Verification items for the finished model (mm, model axes). Face numbers are marked on the shaded views. A direction names the side the tool comes from. Coordinates: 2 decimals unless noted, no trailing zeros. Loops run counter-clockwise (first coordinate to the right, second up) from the corner with the lowest first, then second, coordinate; pieces in that order, holes last. Notation, with made-up numbers: (-1.5, -19.75) - (21.5, -19.75) arc R24 ccw to (21.5, 2.25) - close; hole circle Ø2 at (-33, 10.25). An arc over 180 degrees is marked (long way). Answer as CSV lines item,"result". Start each with the question number.
1. Gauge pin test, flat ends, axial feed: P1, Ø11, axis at x = 14.5, y = 75, coming from the +Z side; P2, Ø6, axis at x = 51.5, z = 40, coming from the +Y side; P3, Ø11, axis at y = 87, z = 4, coming from the -X side. Record the tip position at first contact, or that the pin passes through.
2. Cross-section at B-B (y = 54). Enter the section's corners in (x, z), plus the area to 3 significant figures.
3. Cross-section at A-A (x = 60). State how many separate pieces and enclosed holes the cut face has, plus the area to 3 significant figures.
4. Material ranges on line 1 (X direction, y = 85, z = -20); line 2 (X direction, y = 11, z = -58); line 3 (Z direction, x = 66, y = 67), recorded low to high. Write a range as [from, to].
5. Cross-section at C-C (z = 38). Enter the section's corners in (x, y).
6. Release check for a two-part mould opening along X. For the marked faces 5, 6 and 7 record: pulls with the +X half, pulls with the -X half, needs draft (parallel to the pull), parting line crosses it, or undercut.
7. Set-up check for the marked faces 1, 2, 3 and 4: record each of +Z, -Z, +X, -X, +Y, -Y from which the full face is reachable in a straight line by a thin tool's end or side.
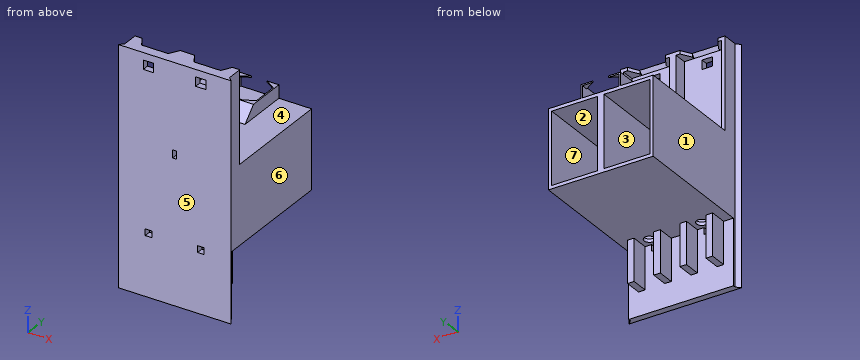
```python
from build123d import *

# Parameters (mm, degrees)
SKETCH1_W                                 = 80
SKETCH1_H                                 = 60
BOSS_EXTRUDE1_DEPTH                       = 100
CUT_EXTRUDE1_START                        = 5
SKETCH2_W                                 = 35
SKETCH2_H                                 = 55
CUT_EXTRUDE1_DEPTH                        = 95
SKETCH3_W                                 = 80
SKETCH3_H                                 = 5
BOSS_EXTRUDE2_DEPTH                       = 70
BOSS_EXTRUDE3_DEPTH                       = 10
SKETCH5_W                                 = 20
SKETCH5_H                                 = 2.5
CUT_EXTRUDE2_DEPTH                        = 7.5
SKETCH6_W                                 = 35
SKETCH6_H                                 = 12
CUT_EXTRUDE4_DEPTH                        = 57.5
CUT_EXTRUDE6_REACH                        = 184.483
SKETCH7_R                                 = 4
SKETCH9_W                                 = 80
SKETCH9_H                                 = 50
BOSS_EXTRUDE4_DEPTH                       = 5
SKETCH13_W                                = 8
SKETCH13_H                                = 7
CUT_EXTRUDE8_BUTTON_HOLES_DEPTH           = 166.90660023
BOSS_EXTRUDE5_OLED_MOUNT_DEPTH            = 10
BOSS_EXTRUDE6_OLED_MOUNT_DEPTH            = 1
BOSS_EXTRUDE7_START                       = -2.5
BOSS_EXTRUDE7_OLED_MOUNT_DEPTH            = 1
BOSS_EXTRUDE8_OLED_MOUNT_DEPTH            = 1
BOSS_EXTRUDE13_OLED_MOUNT_SUPPORT_DEPTH   = 30
CUT_EXTRUDE9_OLED_CABLE_DEPTH             = 10
CUT_EXTRUDE9_OLED_CABLE_DEPTH_BACK        = 154.430766146
SKETCH18_W                                = 3
SKETCH18_H                                = 6
BOSS_EXTRUDE12_OLED_CABLE_GUIDE_REACH     = 162.39
SKETCH20_W                                = 5
SKETCH20_H                                = 5
CUT_EXTRUDE10_SOLENOID_WIRE_HOLE_DEPTH    = 166.90660023
SKETCH21_W                                = 5
SKETCH21_H                                = 32
BOSS_EXTRUDE9_SOLENOID_SIDE_SUPPORT_DEPTH = 13
CHAMFER3_THUMB_SIZE                       = 2.5
CHAMFER5_THUMB_SIZE                       = 4.5
CHAMFER5_THUMB_SIZE2                      = 7.794228634
CHAMFER5_THUMB_PART_2_SIZE                = 4.5
CHAMFER5_THUMB_PART_2_SIZE2               = 7.794228634
CHAMFER5_THUMB_PART_3_SIZE                = 4.5
CHAMFER5_THUMB_PART_3_SIZE2               = 7.794228634
BOSS_EXTRUDE5_GUIDE_DEPTH                 = 180
SKETCH49_W                                = 5
SKETCH49_H                                = 5
BOSS_EXTRUDE14_DEPTH                      = 5
CHAMFER8_SIZE                             = 5


with BuildPart() as part:
    # Sketch1 → Boss-Extrude1 (new body)
    with BuildSketch(Plane(origin=(0, 0, 0), x_dir=(1, 0, 0), z_dir=(0, 1, 0))):
        with Locations((40, 30)):
            Rectangle(SKETCH1_W, SKETCH1_H)
    extrude(amount=BOSS_EXTRUDE1_DEPTH)

    # Sketch2 → Cut-Extrude1 (cut)
    with BuildSketch(Plane(origin=(0, 0, 0), x_dir=(1, 0, 0), z_dir=(0, 1, 0)).offset(CUT_EXTRUDE1_START)):
        with Locations((20, 30)):
            Rectangle(SKETCH2_W, SKETCH2_H)
        with Locations((60, 30)):
            Rectangle(SKETCH2_W, SKETCH2_H)
    extrude(amount=CUT_EXTRUDE1_DEPTH, mode=Mode.SUBTRACT)

    # Sketch3 → Boss-Extrude2 (add)
    with BuildSketch(Plane.XY):
        with Locations((40, 2.5)):
            Rectangle(SKETCH3_W, SKETCH3_H)
    extrude(amount=BOSS_EXTRUDE2_DEPTH)

    # Sketch4 → Boss-Extrude3 (add)
    with BuildSketch(Plane(origin=(0, 5, 0), x_dir=(1, 0, 0), z_dir=(0, 1, 0))):
        Polygon((80, 0), (77.5, 0), (77.5, -67.5), (42.5, -67.5), (42.5, 0), (37.5, 0), (37.5, -67.5), (2.5, -67.5), (2.5, 0), (0, 0), (0, -70), (80, -70), align=None)
    extrude(amount=BOSS_EXTRUDE3_DEPTH)

    # Sketch5 → Cut-Extrude2 (cut)
    with BuildSketch(Plane(origin=(0, 15, 0), x_dir=(1, 0, 0), z_dir=(0, 1, 0))):
        with Locations((20, -68.75)):
            Rectangle(SKETCH5_W, SKETCH5_H)
        with Locations((60, -68.75)):
            Rectangle(SKETCH5_W, SKETCH5_H)
    extrude(amount=-CUT_EXTRUDE2_DEPTH, mode=Mode.SUBTRACT)

    # Sketch6 → Cut-Extrude4 (cut)
    with BuildSketch(Plane.XY):
        with Locations((20, 11)):
            Rectangle(SKETCH6_W, SKETCH6_H)
        with Locations((60, 11)):
            Rectangle(SKETCH6_W, SKETCH6_H)
    extrude(amount=-CUT_EXTRUDE4_DEPTH, mode=Mode.SUBTRACT)

    # Sketch7 → Cut-Extrude6 (cut, up to next)
    with BuildSketch(Plane(origin=(0, 0, -60), x_dir=(-1, 0, 0), z_dir=(0, 0, -1)), mode=Mode.PRIVATE) as cut_extrude6_sk1:
        with Locations((-20, 11.5)):
            Circle(SKETCH7_R)
    cut_extrude6_tool1 = extrude(cut_extrude6_sk1.sketch, amount=-CUT_EXTRUDE6_REACH, mode=Mode.PRIVATE) & part.part
    # Sketch7 → Cut-Extrude6 (cut, up to next)
    with BuildSketch(Plane(origin=(0, 0, -60), x_dir=(-1, 0, 0), z_dir=(0, 0, -1)), mode=Mode.PRIVATE) as cut_extrude6_sk2:
        with Locations((-60, 11.5)):
            Circle(SKETCH7_R)
    cut_extrude6_tool2 = extrude(cut_extrude6_sk2.sketch, amount=-CUT_EXTRUDE6_REACH, mode=Mode.PRIVATE) & part.part
    add(cut_extrude6_tool1.solids().sort_by_distance((20, 11.5, -60))[0], mode=Mode.SUBTRACT)
    add(cut_extrude6_tool2.solids().sort_by_distance((60, 11.5, -60))[0], mode=Mode.SUBTRACT)

    # Sketch9 → Boss-Extrude4 (add)
    with BuildSketch(Plane(origin=(0, 0, 0), x_dir=(1, 0, 0), z_dir=(0, 1, 0))):
        with Locations((40, 85)):
            Rectangle(SKETCH9_W, SKETCH9_H)
    extrude(amount=BOSS_EXTRUDE4_DEPTH)

    # Sketch13 → Cut-Extrude8 (Button Holes) (cut, through all)
    with BuildSketch(Plane(origin=(0, 5, 0), x_dir=(1, 0, 0), z_dir=(0, 1, 0))):
        with Locations((20, -61)):
            Rectangle(SKETCH13_W, SKETCH13_H)
        with Locations((60, -61)):
            Rectangle(SKETCH13_W, SKETCH13_H)
    extrude(amount=-CUT_EXTRUDE8_BUTTON_HOLES_DEPTH, mode=Mode.SUBTRACT)

    # Sketch14 → Boss-Extrude5 (OLED Mount) (add)
    with BuildSketch(Plane.XY):
        Polygon((25, 100), (26, 100), (26, 71), (54, 71), (54, 100), (55, 100), (55, 70), (54, 70), (26, 70), (25, 70), align=None)
    extrude(amount=BOSS_EXTRUDE5_OLED_MOUNT_DEPTH)

    # Sketch15 → Boss-Extrude6 (OLED Mount) (add)
    with BuildSketch(Plane.XY.offset(10)):
        Polygon((26, 71), (34, 71), (26, 75), align=None)
        Polygon((54, 75), (54, 71), (46, 71), align=None)
    extrude(amount=-BOSS_EXTRUDE6_OLED_MOUNT_DEPTH)

    # Sketch15<2> → Boss-Extrude7 (OLED Mount) (add)
    with BuildSketch(Plane.XY.offset(10).offset(BOSS_EXTRUDE7_START)):
        Polygon((26, 71), (34, 71), (26, 75), align=None)
        Polygon((54, 75), (54, 71), (46, 71), align=None)
    extrude(amount=-BOSS_EXTRUDE7_OLED_MOUNT_DEPTH)

    # Sketch17 → Boss-Extrude8 (OLED Mount) (add)
    with BuildSketch(Plane.XY.offset(10)):
        Polygon((54, 95), (54, 100), (46, 100), align=None)
        Polygon((26, 100), (34, 100), (26, 95), align=None)
    extrude(amount=-BOSS_EXTRUDE8_OLED_MOUNT_DEPTH)

    # Sketch32 → Boss-Extrude13 OLED Mount Support) (add)
    with BuildSketch(Plane.ZY.offset(-25)):
        Polygon((0, 70), (10, 70), (0, 60), align=None)
    extrude(amount=-BOSS_EXTRUDE13_OLED_MOUNT_SUPPORT_DEPTH)

    # Sketch18 → Cut-Extrude9 (OLED Cable) (cut, two sides: drawn at the far end of the back side and taken through both)
    with BuildSketch(Plane(origin=(0, 71, 0), x_dir=(1, 0, 0), z_dir=(0, 1, 0)).offset(-CUT_EXTRUDE9_OLED_CABLE_DEPTH_BACK)):
        with Locations((40, -2)):
            Rectangle(SKETCH18_W, SKETCH18_H)
    extrude(amount=CUT_EXTRUDE9_OLED_CABLE_DEPTH + CUT_EXTRUDE9_OLED_CABLE_DEPTH_BACK, mode=Mode.SUBTRACT)

    # Boss-Extrude12 (OLED Cable Guide): up to this plane
    boss_extrude12_oled_cable_guide_end = Plane(origin=(55, 70, 10), z_dir=(0, -0.7071067811865477, 0.7071067811865474))
    # Sketch31 → Boss-Extrude12 (OLED Cable Guide) (add, up to the surface)
    with BuildSketch(Plane(origin=(0, 15, 0), x_dir=(1, 0, 0), z_dir=(0, 1, 0)), mode=Mode.PRIVATE) as boss_extrude12_oled_cable_guide_sk1:
        Polygon((37.5, 0), (38.5, 0), (38.5, -5), (41.5, -5), (41.5, 0), (42.5, 0), (42.5, -7), (37.5, -7), align=None)
    boss_extrude12_oled_cable_guide_tool1 = split(extrude(boss_extrude12_oled_cable_guide_sk1.sketch, amount=BOSS_EXTRUDE12_OLED_CABLE_GUIDE_REACH, mode=Mode.PRIVATE), bisect_by=boss_extrude12_oled_cable_guide_end, keep=Keep.BOTH, mode=Mode.PRIVATE)
    add(boss_extrude12_oled_cable_guide_tool1.solids().sort_by_distance((38, 15, 0.086023))[0])

    # Sketch20 → Cut-Extrude10 (Solenoid Wire Hole) (cut, through all)
    with BuildSketch(Plane(origin=(0, 5, 0), x_dir=(1, 0, 0), z_dir=(0, 1, 0))):
        with Locations((60, 62.5)):
            Rectangle(SKETCH20_W, SKETCH20_H)
        with Locations((20, 62.5)):
            Rectangle(SKETCH20_W, SKETCH20_H)
    extrude(amount=-CUT_EXTRUDE10_SOLENOID_WIRE_HOLE_DEPTH, mode=Mode.SUBTRACT)

    # Sketch21 → Boss-Extrude9 (Solenoid Side Support) (add)
    with BuildSketch(Plane(origin=(0, 5, 0), x_dir=(1, 0, 0), z_dir=(0, 1, 0))):
        with Locations((70, 76)):
            Rectangle(SKETCH21_W, SKETCH21_H)
        with Locations((50, 76)):
            Rectangle(SKETCH21_W, SKETCH21_H)
        with Locations((30, 76)):
            Rectangle(SKETCH21_W, SKETCH21_H)
        with Locations((10, 76)):
            Rectangle(SKETCH21_W, SKETCH21_H)
    extrude(amount=BOSS_EXTRUDE9_SOLENOID_SIDE_SUPPORT_DEPTH)

    # Chamfer3 (Thumb)
    chamfer3_thumb_edges = [part.edges().sort_by_distance(p)[0] for p in [
        (20, 7.5, 67.5),
        (60, 7.5, 67.5),
    ]]
    chamfer(chamfer3_thumb_edges, length=CHAMFER3_THUMB_SIZE - 0.0001)  # a hair under: the kernel refuses the full size

    # Chamfer5 (Thumb)
    chamfer5_thumb_edges = [part.edges().sort_by_distance(p)[0] for p in [
        (70, 15, 68.75),
    ]]
    chamfer5_thumb_side = [part.faces().sort_by_distance(p)[0] for p in [
        (78.266129032, 15, 38.266129032),
    ]]
    chamfer(chamfer5_thumb_edges, length=CHAMFER5_THUMB_SIZE, length2=CHAMFER5_THUMB_SIZE2, reference=chamfer5_thumb_side[0])

    # Chamfer5 (Thumb) part 2
    chamfer5_thumb_part_2_edges = [part.edges().sort_by_distance(p)[0] for p in [
        (50, 15, 68.75),
        (30, 15, 68.75),
    ]]
    chamfer5_thumb_part_2_side = [part.faces().sort_by_distance(p)[0] for p in [
        (40, 15, 41.718085106),
    ]]
    chamfer(chamfer5_thumb_part_2_edges, length=CHAMFER5_THUMB_PART_2_SIZE, length2=CHAMFER5_THUMB_PART_2_SIZE2, reference=chamfer5_thumb_part_2_side[0])

    # Chamfer5 (Thumb) part 3
    chamfer5_thumb_part_3_edges = [part.edges().sort_by_distance(p)[0] for p in [
        (10, 15, 68.75),
    ]]
    chamfer5_thumb_part_3_side = [part.faces().sort_by_distance(p)[0] for p in [
        (1.733870968, 15, 38.266129032),
    ]]
    chamfer(chamfer5_thumb_part_3_edges, length=CHAMFER5_THUMB_PART_3_SIZE, length2=CHAMFER5_THUMB_PART_3_SIZE2, reference=chamfer5_thumb_part_3_side[0])

    # Sketch37 → Boss-Extrude5 (Guide) (add, through all)
    with BuildSketch(Plane.XY.offset(70)):
        Polygon((80, 0), (83, 0), (80, 3), align=None)
        Polygon((0, 0), (-3, 0), (0, 3), align=None)
    extrude(amount=-BOSS_EXTRUDE5_GUIDE_DEPTH)

    # Sketch49 → Boss-Extrude14 (add)
    with BuildSketch(Plane(origin=(0, 15, 0), x_dir=(1, 0, 0), z_dir=(0, 1, 0))):
        with Locations((40, -9.5)):
            Rectangle(SKETCH49_W, SKETCH49_H)
    extrude(amount=BOSS_EXTRUDE14_DEPTH)

    # Chamfer8
    chamfer8_edges = [part.edges().sort_by_distance(p)[0] for p in [
        (40, 20, 12),
    ]]
    chamfer(chamfer8_edges, length=CHAMFER8_SIZE - 0.0001)  # a hair under: the kernel refuses the full size


solid = part.part
```
Values follow:
1,P1,"stops at z = 0"
1,P2,"stops at y = 5"
1,P3,"stops at x = 0"
2,outline,"(0, -60) - (80, -60) - (80, 0) - (42.5, 0) - (42.5, 7) - (37.5, 7) - (37.5, 0) - (0, 0) - close; hole (2.5, -57.5) - (37.5, -57.5) - (37.5, -2.5) - (2.5, -2.5) - close; hole (38.5, -1) - (41.5, -1) - (41.5, 5) - (38.5, 5) - close; hole (42.5, -57.5) - (77.5, -57.5) - (77.5, -2.5) - (42.5, -2.5) - close"
2,area,"967 mm²"
3,separate pieces,"5"
3,enclosed holes,"0"
3,area,"1,270 mm²"
4,line 1,"x = [0, 2.5], [37.5, 42.5], [77.5, 80]"
4,line 2,"x = [0, 16.03], [23.97, 56.03], [63.97, 80]"
4,line 3,"z = [-60, -57.5], [-2.5, 0]"
5,outline,"(-3, 0) - (83, 0) - (80, 3) - (80, 15) - (77.5, 15) - (77.5, 5) - (42.5, 5) - (42.5, 15) - (37.5, 15) - (37.5, 5) - (2.5, 5) - (2.5, 15) - (0, 15) - (0, 3) - close"
6,face 5,"needs draft"
6,face 6,"pulls with the +X half"
6,face 7,"undercut"
7,face 1,"+Z, -Z, -X, +Y"
7,face 2,"+Y"
7,face 3,"none"
7,face 4,"+Z, +X"
